from build123d import *

# Parameters (mm, degrees)
SKETCH_1_R          = 127.5
EXTRUDE_1_DEPTH     = 6
SKETCH_2_R          = 127.5
SKETCH_2_R_2        = 122.5
EXTRUDE_2_DEPTH     = 220
SKETCH_3_R          = 10
CUT_EXTRUDE_1_DEPTH = 200
FILLET_1_R          = 10
CHAMFER_1_SIZE      = 8
FILLET_2_R          = 1
CHAMFER_2_SIZE      = 1
FILLET_3_R          = 1


with BuildPart() as part:
    # 草图1 → 凸台-拉伸1 (new body)
    with BuildSketch(Plane(origin=(0, 0, 0), x_dir=(1, 0, 0), z_dir=(0, 1, 0))):
        with Locations(Location((0, 0, 0), (0, 0, 270))):
            Circle(SKETCH_1_R)
    extrude(amount=EXTRUDE_1_DEPTH)

    # 草图2 → 凸台-拉伸2 (add)
    with BuildSketch(Plane(origin=(0, 6, 0), x_dir=(1, 0, 0), z_dir=(0, 1, 0))):
        with Locations(Location((0, 0, 0), (0, 0, 270))):
            Circle(SKETCH_2_R)
        with Locations(Location((0, 0, 0), (0, 0, 270))):
            Circle(SKETCH_2_R_2, mode=Mode.SUBTRACT)
    extrude(amount=EXTRUDE_2_DEPTH)

    # 草图3 → 切除-拉伸1 (cut)
    with BuildSketch(Plane(origin=(0, 6, 0), x_dir=(1, 0, 0), z_dir=(0, 1, 0))):
        with Locations(Location((0, 0, 0), (0, 0, 270))):
            Circle(SKETCH_3_R)
    extrude(amount=-CUT_EXTRUDE_1_DEPTH, mode=Mode.SUBTRACT)

    # 圆角1
    fillet_1_edges = [part.edges().sort_by_distance(p)[0] for p in [
        (0, 6, -122.5),
    ]]
    fillet(fillet_1_edges, radius=FILLET_1_R)

    # 倒角1
    chamfer_1_edges = [part.edges().sort_by_distance(p)[0] for p in [
        (0, 0, -127.5),
    ]]
    chamfer(chamfer_1_edges, length=CHAMFER_1_SIZE)

    # 圆角2
    fillet_2_edges = [part.edges().sort_by_distance(p)[0] for p in [
        (0, 226, -127.5),
        (0, 226, -122.5),
    ]]
    fillet(fillet_2_edges, radius=FILLET_2_R)

    # 倒角2
    chamfer_2_edges = [part.edges().sort_by_distance(p)[0] for p in [
        (0, 0, -10),
    ]]
    chamfer(chamfer_2_edges, length=CHAMFER_2_SIZE)

    # 圆角3
    fillet_3_edges = [part.edges().sort_by_distance(p)[0] for p in [
        (0, 6, -10),
    ]]
    fillet(fillet_3_edges, radius=FILLET_3_R)


solid = part.part
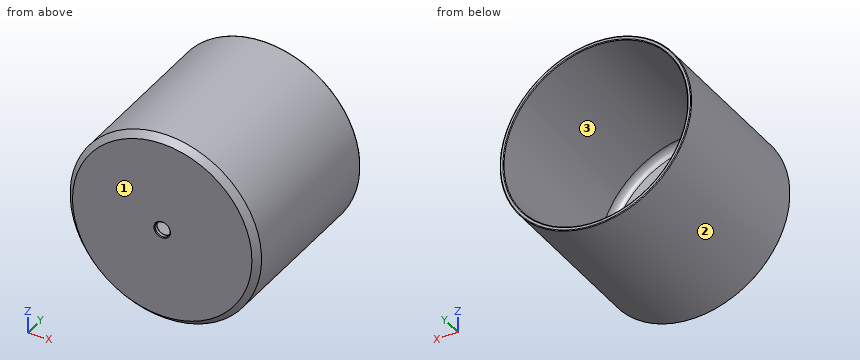
Can you work these out from the model? Positions are in its coordinate system, mm. Face numbers are marked on the shaded views. Coordinates: 2 decimals unless noted, no trailing zeros. Loops run counter-clockwise (first coordinate to the right, second up) from the corner with the lowest first, then second, coordinate; pieces in that order, holes last. Notation, with made-up numbers: (26.5, 0.5) - (66.5, 0.5) arc R29 cw to (66.5, 37.5) - close; hole circle Ø1 at (74.25, 74.25). An arc over 180 degrees is marked (long way). Answer as a JSON object with one key per item and string values. Group by question number.
Item 1: If we section it at A-A (z = 0): List the corners of the cut face in (x, y) for me, plus the area to 3 significant figures.
Item 2: If I drill on L1, parallel to X at y = 181, z = 0; L2, parallel to Z at x = 3.5, y = 192; L3, parallel to Z at x = 2.5, y = 76, over which ranges is the centre line in solid material (lowest first)? Write a range as from..to.
Item 3: If we section it at C-C (y = 177.5): List the corners of the cut face in (x, z) for me, plus the area to 3 significant figures.
Item 4: If we mould it in two halves opening along X, with no side actions, what happens to the marked faces 1, 2 and 3? For each: released by +X, released by -X, zero draft, split by the parting line, or undercut.
Item 5: If we section it at B-B (x = 0): List the corners of the cut face in (y, z) for me, plus the area to 3 significant figures.
Item 6: For pin 1 (3 mm diameter, centred on x = 18.5, y = 48.5, fed in from +Z); pin 2 (4 mm diameter, centred on x = -101.5, y = 176, fed in from +Z); pin 3 (10 mm diameter, centred on x = -65, y = 137.5, fed in from -Z), each with a flat end and sliding along its axis, tell me the tip position at first contact or that it passes through.
Returned:
{
 "1": {"outline": "(-127.5, 8) - (-119.5, 0) - (-11, 0) - (-10, 1) - (-10, 5) arc R1 ccw to (-11, 6) - (-112.5, 6) arc R10 cw to (-122.5, 16) - (-122.5, 225) arc R1 ccw to (-123.5, 226) - (-126.5, 226) arc R1 ccw to (-127.5, 225) - close; (10, 1) - (11, 0) - (119.5, 0) - (127.5, 8) - (127.5, 225) arc R1 ccw to (126.5, 226) - (123.5, 226) arc R1 ccw to (122.5, 225) - (122.5, 16) arc R10 cw to (112.5, 6) - (11, 6) arc R1 ccw to (10, 5) - close", "area": "3,590 mm²"},
 "2": {"L1": "x = -127.5..-122.5, 122.5..127.5", "L2": "z = -127.45..-122.45, 122.45..127.45", "L3": "z = -127.48..-122.47, 122.47..127.48"},
 "3": {"outline": "circle Ø255 at (0, 0); hole circle Ø245 at (0, 0)", "area": "3,930 mm²"},
 "4": {"face 1": "zero draft", "face 2": "split by the parting line", "face 3": "undercut"},
 "5": {"outline": "(0, -119.5) - (8, -127.5) - (225, -127.5) arc R1 ccw to (226, -126.5) - (226, -123.5) arc R1 ccw to (225, -122.5) - (16, -122.5) arc R10 cw to (6, -112.5) - (6, -11) arc R1 ccw to (5, -10) - (1, -10) - (0, -11) - close; (0, 11) - (1, 10) - (5, 10) arc R1 ccw to (6, 11) - (6, 112.5) arc R10 cw to (16, 122.5) - (225, 122.5) arc R1 ccw to (226, 123.5) - (226, 126.5) arc R1 ccw to (225, 127.5) - (8, 127.5) - (0, 119.5) - close", "area": "3,590 mm²"},
 "6": {"pin 1": "stops at z = 126.36", "pin 2": "stops at z = 79.72", "pin 3": "stops at z = -112.5"}
}
